Drawing for the job (mm, zero at the part's lowest x, y, z). A direction names the side the tool comes from. Coordinates: 2 decimals unless noted, no trailing zeros. Order: outer loops, then holes, each group sorted by start corner. A loop starts at its lowest first (then second) coordinate and runs counter-clockwise, first axis right, second up.
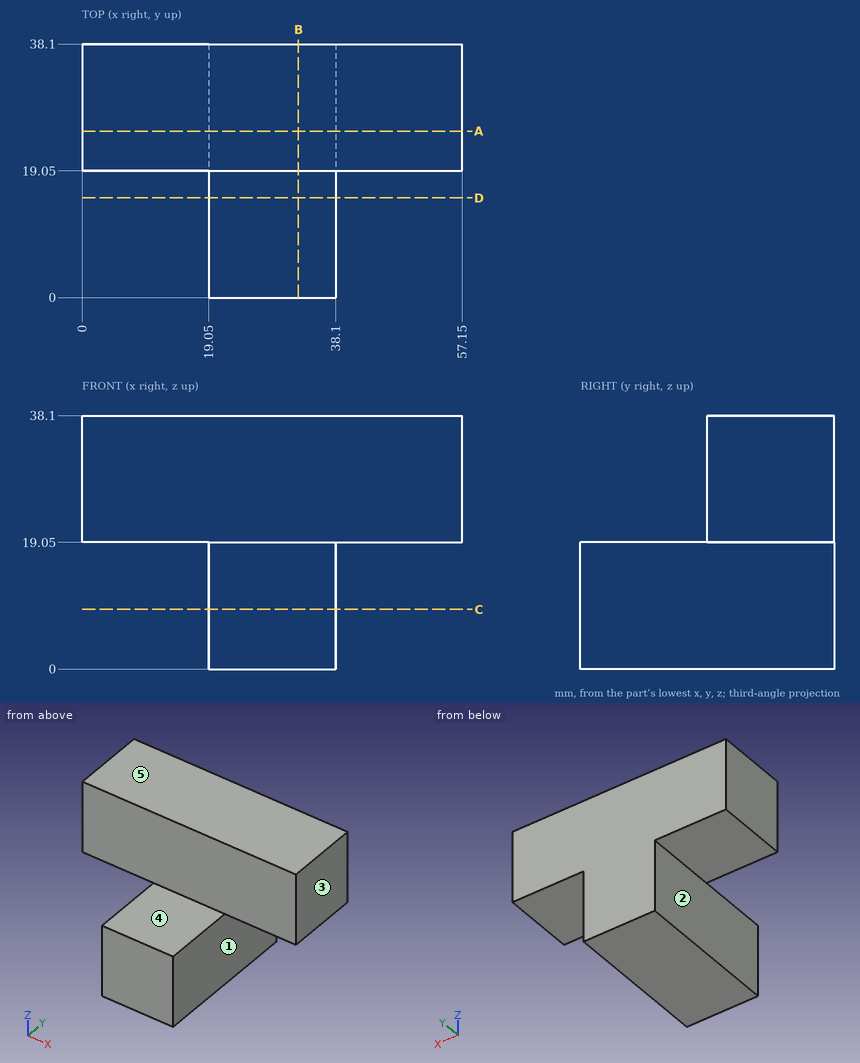
1) Slice it at A-A (y = 25). List the corners of the cut face in (x, z), plus the area to 3 significant figures.
2) Slice it at C-C (z = 9). List the corners of the cut face in (x, y).
3) Slice it at B-B (x = 32.5). List the corners of the cut face in (y, z).
4) Slice it at D-D (y = 15). List the corners of the cut face in (x, z), plus the area to 3 significant figures.
5) Drill centre lines: probe 1 along X at (y, z) = (4, 18); probe 2 along Z at (x, y) = (20, 3). Where is each one in solid material? Low to high.
6) Which spindle directions (+Z, -Z, +X, -X, +Y, -Y) get a long thin tool onto all of the face, cutting with end or side? Do the marked faces 1, 2, 3, 4 and 5. Say none if no direction does.
7) Pin check, flat tips, straight feed: P1, Ø1.5, axis at y = 10.5, z = 6.5, coming from the -X side; P2, Ø15, axis at x = 11.5, y = 26, coming from the -Z side; P3, Ø21, axis at y = 26.5, z = 6, coming from the +X side. Stop position of each tip, or through.
Worked out:
1. outline: (0, 19.05) - (19.05, 19.05) - (19.05, 0) - (38.1, 0) - (38.1, 19.05) - (57.15, 19.05) - (57.15, 38.1) - (0, 38.1) - close
1. area: 1,450 mm2
2. outline: (19.05, 0) - (38.1, 0) - (38.1, 38.1) - (19.05, 38.1) - close
3. outline: (0, 0) - (38.1, 0) - (38.1, 38.1) - (19.05, 38.1) - (19.05, 19.05) - (0, 19.05) - close
4. outline: (19.05, 0) - (38.1, 0) - (38.1, 19.05) - (19.05, 19.05) - close
4. area: 363 mm2
5. probe 1: x = 19.05 to 38.1
5. probe 2: z = 0 to 19.05
6. face 1: -Z, +X, +Y, -Y
6. face 2: -Z, -X, +Y, -Y
6. face 3: +Z, -Z, +X, +Y, -Y
6. face 4: +Z, +X, -X, -Y
6. face 5: +Z, +X, -X, +Y, -Y
7. P1: stops at x = 19.05
7. P2: stops at z = 19.05
7. P3: stops at x = 38.1
